from build123d import *

# Parameters (mm, degrees)
F0_W     = 6.5
F0_H     = 9
F2_DEPTH = 0.6
F1_W     = 5.5
F1_H     = 8
F3_DEPTH = 0.6
F4_R     = 0.2


with BuildPart() as f2:
    # F0 (on Top) → F2 (new body)
    with BuildSketch(Plane.XY):
        with Locations((3.25, 4.5)):
            Rectangle(F0_W, F0_H)
    extrude(amount=-F2_DEPTH)

    # F1 (on face) → F3 (join)
    with BuildSketch(Plane.XY):
        with Locations((3.25, 4.5)):
            Rectangle(F1_W, F1_H)
    extrude(amount=F3_DEPTH)

    # F4
    f4_edges = [f2.edges().sort_by_distance(p)[0] for p in [
        (0.5, 4.5, 0.6),
        (3.25, 0.5, 0.6),
        (6, 4.5, 0.6),
        (3.25, 8.5, 0.6),
    ]]
    fillet(f4_edges, radius=F4_R)


solid = f2.part
Read the model definition and answer for the solid it produces. Units are mm, in the model's axes. Round coordinates to 2 decimals unless told otherwise and drop trailing zeros. Write each loop counter-clockwise with the first axis right and the second up, starting at its lowest first coordinate (ties: lowest second). Pieces come first, ordered by that corner, then holes. Notation, with made-up numbers: (15, 77.25) - (39, 77.25) arc R28 cw to (39, 112.25) - close; hole circle Ø9 at (-34.5, 49.25). An arc over 180 degrees is marked (long way). Use a Markdown table: item, result.
(1) The part is cut by section B-B (y = 8). Write down the section's boundary in (x, z).
Reported:
| item | result |
|---|---|
| outline | (0, -0.6) - (6.5, -0.6) - (6.5, 0) - (6, 0) - (6, 0.4) arc R0.2 ccw to (5.8, 0.6) - (0.7, 0.6) arc R0.2 ccw to (0.5, 0.4) - (0.5, 0) - (0, 0) - close |
(2) Straight lines are drawn through the part: line 1 along X through (y, z) = (1.5, 0.25); line 2 along Y through (x, z) = (3, 0.15); line 3 along Z through (x, y) = (6.25, 7.25). For each, find the intervals that lie inside material, in ascending order. Write a range as [from, to].
Reported:
| item | result |
|---|---|
| line 1 | [0.5, 6] |
| line 2 | [0.5, 8.5] |
| line 3 | [-0.6, 0] |
(3) The part is cut by section C-C (z = 0.15). Write down the section's boundary in (x, y).
Reported:
| item | result |
|---|---|
| outline | (0.5, 0.5) - (6, 0.5) - (6, 8.5) - (0.5, 8.5) - close |
(4) The part is cut by section A-A (x = 1). Write down the section's boundary in (y, z), then the cut area to 3 significant figures.
Reported:
| item | result |
|---|---|
| outline | (0, -0.6) - (9, -0.6) - (9, 0) - (8.5, 0) - (8.5, 0.4) arc R0.2 ccw to (8.3, 0.6) - (0.7, 0.6) arc R0.2 ccw to (0.5, 0.4) - (0.5, 0) - (0, 0) - close |
| area | 10.2 mm2 |
(5) The mould has two halves that part along Z. Classify faces 1 (the flat face through (3, 5, 0.6)), 2 (the flat face through (3, 5, -0.6)): released by +Z, released by -Z, zero draft, split by the parting line, or undercut.
Reported:
| item | result |
|---|---|
| face 1 | released by +Z |
| face 2 | released by -Z |
(6) The part is cut by section D-D (x = 6.25). Write down the section's boundary in (y, z), then the cut area to 3 significant figures.
Reported:
| item | result |
|---|---|
| outline | (0, -0.6) - (9, -0.6) - (9, 0) - (0, 0) - close |
| area | 5.40 mm2 |
